Design review of the part built by this model. Coordinates are the model's own, in mm. Face numbers are marked on the shaded views. A direction names the side the tool comes from. Coordinates: 2 decimals unless noted, no trailing zeros. Write each loop counter-clockwise with the first axis right and the second up, starting at its lowest first coordinate (ties: lowest second). Pieces come first, ordered by that corner, then holes. Notation, with made-up numbers: (86, 77) - (93, 77) arc R8 cw to (93, 82) - close; hole circle Ø9 at (79, -15). An arc over 180 degrees is marked (long way). One line per item, written item: value.
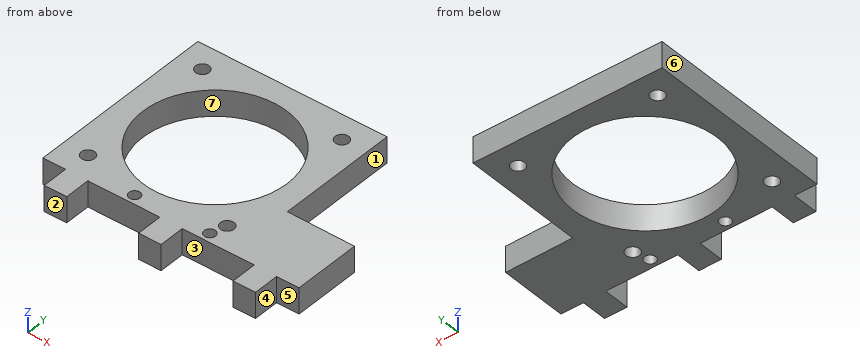
from build123d import *

# Parameters (mm, degrees)
SKETCH1_R           = 16
SKETCH1_R_2         = 1.25
SKETCH1_R_3         = 1.5
BOSS_EXTRUDE1_DEPTH = 5.72


with BuildPart() as part:
    # Sketch1 → Boss-Extrude1 (new body)
    with BuildSketch(Plane.XY):
        Polygon((9.38, 32.147938931), (9.38, 5.147938931), (24.38, 5), (24.38, -10), (19.38, -10), (19.38, -15.72), (14.38, -15.72), (14.38, -9.950687023), (-1.62, -9.950687023), (-1.62, -15.670687023), (-6.62, -15.670687023), (-6.62, -9.901374046), (-22.62, -9.901374046), (-22.62, -15.621374046), (-27.62, -15.621374046), (-27.62, -9.852061069), (-32.62, -9.852061069), (-32.62, 32.147938931), align=None)
        with Locations((-11.62, 11.147938931)):
            Circle(SKETCH1_R, mode=Mode.SUBTRACT)
        with Locations((2.88, -7.950687023)):
            Circle(SKETCH1_R_2, mode=Mode.SUBTRACT)
        with Locations((-13.87, -7.901374046)):
            Circle(SKETCH1_R_2, mode=Mode.SUBTRACT)
        with Locations((3.879843111, -4.450687023)):
            Circle(SKETCH1_R_3, mode=Mode.SUBTRACT)
        with Locations((-27.12, -4.352061069)):
            Circle(SKETCH1_R_3, mode=Mode.SUBTRACT)
        with Locations((-27.12, 26.647938931)):
            Circle(SKETCH1_R_3, mode=Mode.SUBTRACT)
        with Locations((3.88, 26.647938931)):
            Circle(SKETCH1_R_3, mode=Mode.SUBTRACT)
    extrude(amount=BOSS_EXTRUDE1_DEPTH)


solid = part.part
1. For the marked faces 1, 2, 3 and 4, list the 3-axis set-ups (+Z, -Z, +X, -X, +Y, -Y) from which the entire face can be reached by the end or side of a thin tool; tool diameter is ignored.
Answer block:
face 1: +Z, -Z, +X, +Y
face 2: +Z, -Z, -X, -Y
face 3: +Z, -Z, -Y
face 4: +Z, -Z, +X, -Y
2. Insertion check: pin 1 Ø2.5 at (x, z) = (-29, 2) entering from -Y; pin 2 Ø1.5 at (x, z) = (-3.5, 2) entering from -Y; pin 3 Ø2.5 at (x, z) = (-26.5, 4) entering from -Y; pin 4 Ø12 at (x, y) = (17, 13.5) entering from +Z. Each pin has a flat end and moves straight along its axis. Give the tip position at first contact, or say it passes through.
Answer block:
pin 1: stops at y = -9.85
pin 2: stops at y = -15.67
pin 3: stops at y = -15.62
pin 4: passes through
3. Mouldability with a two-part tool opening along Y and no side actions: class the marked faces 5, 6 and 7 as released by +Y, released by -Y, zero draft, split by the parting line, or undercut.
Answer block:
face 5: released by -Y
face 6: zero draft
face 7: undercut
4. Consider section B-B, the plane x = -13.87. Write out the cut boundary in (y, z).
Answer block:
outline: (-9.9, 0) - (-9.15, 0) - (-9.15, 5.72) - (-9.9, 5.72) - close; (-6.65, 0) - (-4.69, 0) - (-4.69, 5.72) - (-6.65, 5.72) - close; (26.99, 0) - (32.15, 0) - (32.15, 5.72) - (26.99, 5.72) - close
5. Consider section C-C, the plane z = 2.95. Write out the cut boundary in (x, y).
Answer block:
outline: (-32.62, -9.85) - (-27.62, -9.85) - (-27.62, -15.62) - (-22.62, -15.62) - (-22.62, -9.9) - (-6.62, -9.9) - (-6.62, -15.67) - (-1.62, -15.67) - (-1.62, -9.95) - (14.38, -9.95) - (14.38, -15.72) - (19.38, -15.72) - (19.38, -10) - (24.38, -10) - (24.38, 5) - (9.38, 5.15) - (9.38, 32.15) - (-32.62, 32.15) - close; hole circle Ø3 at (-27.12, -4.35); hole circle Ø3 at (-27.12, 26.65); hole circle Ø32 at (-11.62, 11.15); hole circle Ø2.5 at (-13.87, -7.9); hole circle Ø2.5 at (2.88, -7.95); hole circle Ø3 at (3.88, -4.45); hole circle Ø3 at (3.88, 26.65)
6. Consider section D-D, the plane x = 3.5. Write out the cut boundary in (y, z), then the cut area to 3 significant figures.
Answer block:
outline: (-9.95, 0) - (-9.04, 0) - (-9.04, 5.72) - (-9.95, 5.72) - close; (-6.87, 0) - (-5.9, 0) - (-5.9, 5.72) - (-6.87, 5.72) - close; (-3, 0) - (5.91, 0) - (5.91, 5.72) - (-3, 5.72) - close; (16.38, 0) - (25.2, 0) - (25.2, 5.72) - (16.38, 5.72) - close; (28.1, 0) - (32.15, 0) - (32.15, 5.72) - (28.1, 5.72) - close
area: 135 mm^2
7. Consider section A-A, the plane y = 16. Write out the cut boundary in (x, z), then the cut area to 3 significant figures.
Answer block:
outline: (-32.62, 0) - (-26.87, 0) - (-26.87, 5.72) - (-32.62, 5.72) - close; (3.63, 0) - (9.38, 0) - (9.38, 5.72) - (3.63, 5.72) - close
area: 65.8 mm^2
8. Wall thickness on line 1 along X through (y, z) = (-10.5, 1.45); line 2 along Y through (x, z) = (2.88, 3.5); line 3 along X through (y, z) = (-3.5, 3.55): over which ranges is each line inside the solid? List them lowest first.
Answer block:
line 1: x = -27.62 to -22.62, -6.62 to -1.62, 14.38 to 19.38
line 2: y = -9.95 to -9.2, -6.7 to -5.57, -3.33 to 4.38, 17.91 to 25.53, 27.77 to 32.15
line 3: x = -32.62 to -28.35, -25.89 to -18.06, -5.18 to 2.72, 5.04 to 24.38
